Verification items for the finished model (mm, model axes). Round coordinates to 2 decimals unless told otherwise and drop trailing zeros. Write each loop counter-clockwise with the first axis right and the second up, starting at its lowest first coordinate (ties: lowest second). Pieces come first, ordered by that corner, then holes. Notation, with made-up numbers: M 61.25,23 L 80.25,23 A33 cw 80.25,56 Z; hole C 0,56.25 d1. An arc over 180 degrees is marked long. One line per item, written item: value. Start each with the question number.
from build123d import *

# Parameters (mm, degrees)
MODEL_W                 = 3
MODEL_H                 = 5
SALIENTE_EXTRUIR1_DEPTH = 3


with BuildPart() as part:
    # Model → Saliente-Extruir1 (new body)
    with BuildSketch(Plane.XY):
        with BuildLine():
            Line((25.823008531, 25.328827472), (25.823008531, -27.332866004))
            ThreePointArc((25.823008531, -27.332866004), (28.747771663, -34.399762301), (35.811213184, -37.332859048))
            Line((35.811213184, -37.332859048), (81.813268997, -37.378641912))
            ThreePointArc((81.813268997, -37.378641912), (88.89063275, -34.453157454), (91.823009601, -27.378646656))
            Line((91.823009601, -27.378646656), (91.823009601, 34.821697163))
            ThreePointArc((91.823009601, 34.821697163), (88.685239194, 39.45821871), (83.197638532, 38.349537442))
            ThreePointArc((83.197638532, 38.349537442), (83.091891778, 38.246548616), (82.983150977, 38.146726212))
            ThreePointArc((82.983150977, 38.146726212), (79.158392414, 35.809046345), (74.756507073, 34.962328761))
            ThreePointArc((74.756507073, 34.962328761), (73.700057315, 35.063620335), (72.68878473, 35.38560455))
            ThreePointArc((72.68878473, 35.38560455), (68.069225879, 37.194690132), (63.316100845, 38.616279747))
            ThreePointArc((63.316100845, 38.616279747), (62.485957107, 38.754544477), (61.644382862, 38.751619998))
            ThreePointArc((61.644382862, 38.751619998), (58.215145594, 37.688534886), (55.531115502, 35.304043186))
            ThreePointArc((55.531115502, 35.304043186), (54.958944511, 34.649794571), (54.282120522, 34.104514662))
            ThreePointArc((54.282120522, 34.104514662), (50.140040935, 32.758182229), (45.908966143, 33.791352311))
            ThreePointArc((45.908966143, 33.791352311), (45.116243353, 34.349525285), (44.446145174, 35.050192768))
            ThreePointArc((44.446145174, 35.050192768), (41.500295, 38.141911881), (38.022338936, 40.619931641))
            ThreePointArc((38.022338936, 40.619931641), (35.993879777, 41.16016146), (33.903505077, 40.96825411))
            ThreePointArc((33.903505077, 40.96825411), (29.987740451, 39.437981004), (26.890761417, 36.594801579))
            ThreePointArc((26.890761417, 36.594801579), (26.097480223, 35.140352586), (25.823008531, 33.506528172))
            Line((25.823008531, 33.506528172), (25.823008531, 25.328827472))
        make_face()
        with Locations((56.123009601, -12.898202125)):
            Rectangle(MODEL_W, MODEL_H, mode=Mode.SUBTRACT)
        with Locations((46.123009601, -12.898202125)):
            Rectangle(MODEL_W, MODEL_H, mode=Mode.SUBTRACT)
        with Locations((56.123009601, -27.898202125)):
            Rectangle(MODEL_W, MODEL_H, mode=Mode.SUBTRACT)
        with Locations((46.123009601, -27.898202125)):
            Rectangle(MODEL_W, MODEL_H, mode=Mode.SUBTRACT)
        with BuildLine():
            ThreePointArc((31.891647008, 14.698529627), (34.737479764, 17.894903167), (34.068174805, 22.121911417))
            ThreePointArc((34.068174805, 22.121911417), (33.201238031, 23.883836719), (32.862791652, 25.818110274))
            ThreePointArc((32.862791652, 25.818110274), (33.159875497, 29.564217988), (35.254372097, 32.684260585))
            ThreePointArc((35.254372097, 32.684260585), (36.97332261, 33.76093452), (38.880316643, 33.069999366))
            ThreePointArc((38.880316643, 33.069999366), (39.303180243, 22.39412756), (31.891647008, 14.698529627))
        make_face(mode=Mode.SUBTRACT)
        with BuildLine():
            ThreePointArc((60.669464902, 33.72846753), (58.153624192, 33.64814712), (56.308435323, 31.936077063))
            ThreePointArc((56.308435323, 31.936077063), (56.034810359, 26.550644681), (59.015292929, 22.056818226))
            ThreePointArc((59.015292929, 22.056818226), (62.490702694, 27.517307494), (60.669464902, 33.72846753))
        make_face(mode=Mode.SUBTRACT)
        with BuildLine():
            ThreePointArc((87.974912144, 32.931323036), (86.39007686, 33.704958001), (84.750501033, 33.055338848))
            ThreePointArc((84.750501033, 33.055338848), (82.332342702, 29.830877737), (82.3321927, 25.800413849))
            ThreePointArc((82.3321927, 25.800413849), (85.598214893, 24.80893095), (88.439971438, 26.699528486))
            ThreePointArc((88.439971438, 26.699528486), (88.820060436, 29.86114357), (87.974912144, 32.931323036))
        make_face(mode=Mode.SUBTRACT)
    extrude(amount=SALIENTE_EXTRUIR1_DEPTH)


solid = part.part
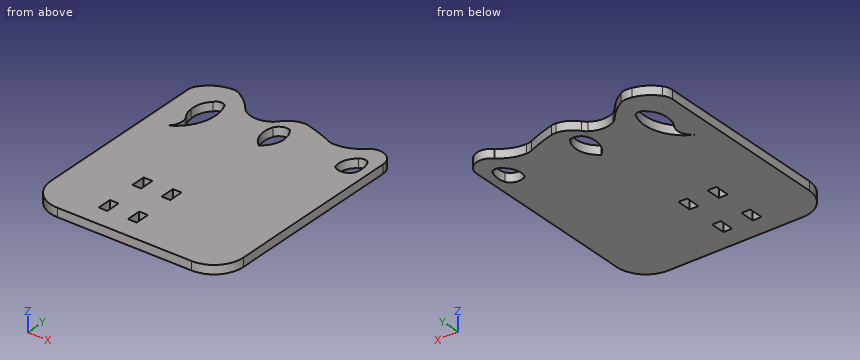
1) Cross-section at C-C (x = 76). Record the boundary of the cut face in (y, z), then the cut area to 3 significant figures.
2) Thickness scan on line 1 (Y direction, x = 46, z = 0.55); line 2 (Y direction, x = 49.5, z = 2.85); line 3 (X direction, y = 20.5, z = 1.8). Record the ranges inside material, lowest first.
3) Cross-section at A-A (z = 2.55). State how many separate pieces and enclosed holes the cut face has, then the cut area to 3 significant figures.
4) Cross-section at B-B (x = 51.5). Record the boundary of the cut face in (y, z).
5) Gauge pin test, flat ends, axial feed: pin 1 Ø1.5 at (x, z) = (56, 1) entering from +Y; pin 2 Ø0.9 at (x, z) = (56, 2) entering from -Y; pin 3 Ø5 at (x, y) = (78, 13) entering from -Z; pin 4 Ø0.9 at (y, z) = (-29, 1.5) entering from -X. Record the tip position at first contact, or that the pin passes through.
Results below:
1. outline: M -37.37,0 L 35.04,0 L 35.04,3 L -37.37,3 Z
1. area: 217 mm²
2. line 1: y = -37.34 to -30.4, -25.4 to -15.4, -10.4 to 33.74
2. line 2: y = -37.35 to 32.76
2. line 3: x = 25.82 to 34.79, 38.41 to 91.82
3. separate pieces: 1
3. enclosed holes: 7
3. area: 4,620 mm²
4. outline: M -37.35,0 L 32.93,0 L 32.93,3 L -37.35,3 Z
5. pin 1: stops at y = 36.64
5. pin 2: stops at y = -37.35
5. pin 3: stops at z = 0
5. pin 4: stops at x = 25.9
